For this review, take the finished solid that the model builds, in its own axes (mm). Face numbers are marked on the shaded views. A direction names the side the tool comes from. Round coordinates to 2 decimals unless told otherwise and drop trailing zeros. Order: outer loops, then holes, each group sorted by start corner. A loop starts at its lowest first (then second) coordinate and runs counter-clockwise, first axis right, second up. Notation, with made-up numbers: M 27,-30.5 L 78,-30.5 A16 cw 78,-15.5 Z; hole C 42.5,60.25 d1. An arc over 180 degrees is marked long. Answer as a JSON object with one key per item and string values.
Autodesk Inventor part; units mm, degrees
ref_plane "YZ Plane" through (0, 0, 0) normal (1, 0, 0) x (0, 1, 0)
ref_plane "XZ Plane" through (0, 0, 0) normal (0, 1, 0) x (-1, 0, 0)
ref_plane "XY Plane" through (0, 0, 0) normal (0, 0, 1) x (1, 0, 0)
sketch "Эскиз1" plane through (0, 0, 0) normal (0, 1, 0) x (-1, 0, 0)
  circle A0 centre (0, 0) radius 4.6
  dimension "d0" = 9.2
extrude "Выдавливание1" add sketch "Эскиз1" along normal blind 2.5
sketch "Эскиз2" plane through (0, 2.5, 0) normal (0, 1, 0) x (1, 0, 0)
  circle A0 centre (0, 0) radius 2.5
  dimension "d3" = 5
extrude "Выдавливание2" add sketch "Эскиз2" along normal blind 10
chamfer "Фаска1" distance 2.1 angle 45 1 edges at (4.6, 2.5, 0)
thread "Резьба1"
chamfer "Фаска2" distance 0.5 angle 45 1 edges at (-2.5, 12.5, 0)
sketch "Эскиз3" plane through (0, 0, 0) normal (0, -1, 0) x (1, 0, 0)
  line L0 (-6.5735, -0.75) -> (6.5735, -0.75)
  line L1 (6.5735, -0.75) -> (6.5735, 0.75)
  line L2 (6.5735, 0.75) -> (-6.5735, 0.75)
  line L3 (-6.5735, 0.75) -> (-6.5735, -0.75)
  line L4 (-6.5735, -0.75) -> (6.5735, 0.75) construction
  line L5 (6.5735, -0.75) -> (-6.5735, 0.75) construction
  point P0 (0, 0)
  dimension "d14" = 1.5
extrude "Выдавливание3" cut sketch "Эскиз3" against normal blind 1
properties part number "Винт М5х10 с потайной головкой" material "Сталь"
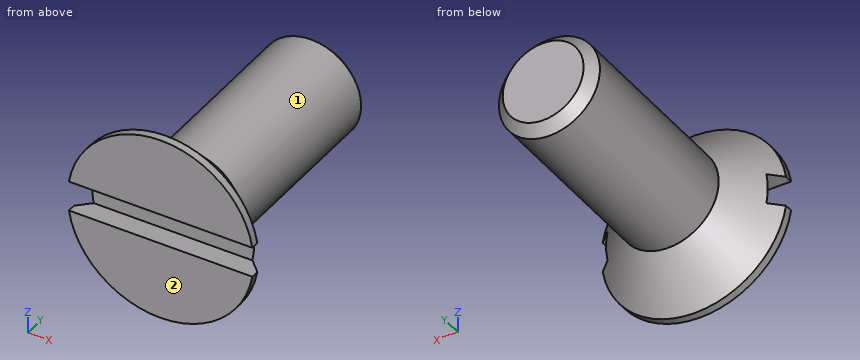
1) Machinability: for the marked faces 1 and 2, which of the approach directions +Z, -Z, +X, -X, +Y, -Y give a long, thin tool a straight path to every point of the face, cutting with its end or side? Answer none if there is none.
Geometry check:
{"face 1": "+Y", "face 2": "+Z, -Z, +X, -X, -Y"}
2) For L1, parallel to X at y = 9.5, z = -1.5; L2, parallel to Y at x = 1, z = -2, list the stretches that pass through material, from the lowest coordinate up.
Geometry check:
{"L1": "x = -2 to 2", "L2": "y = 0 to 12.26"}
3) Insertion check: P1, Ø1, axis at x = -3, z = 1, coming from the +Y side; P2, Ø5, axis at y = 7.5, z = 3, coming from the -X side; P3, Ø4, axis at y = 10, z = 0.5, coming from the -X side. Each pin has a flat end and moves straight along its axis. Give the tip position at first contact, or say it passes through.
Geometry check:
{"P1": "stops at y = 2.34", "P2": "stops at x = -2.45", "P3": "stops at x = -2.5"}
4) Add section C-C on y = 10.25. State the section outline as (x, z) points.
Geometry check:
{"outline": "C 0,0 d5"}
